from build123d import *

# Parameters (mm, degrees)
SKETCH1_W              = 44
SKETCH1_H              = 320
BASE_FLANGE1_DEPTH     = 1.2
SKETCHED_START         = -22
SKETCHED_BEND1_DEPTH   = 44
SKETCHED_BEND1_2_DEPTH = 44
SKETCH7_R              = 4.5
CUT_EXTRUDE1_DEPTH     = 10
SKETCH8_R              = 4
CUT_EXTRUDE2_DEPTH     = 10


# Read off the part's stored shape, not the designer's step: Sketched Bend1
# Sheet-metal steps are written as plain solids
with BuildPart() as part:
    # Sketch1 → Base-Flange1 (new body)
    with BuildSketch(Plane(origin=(0, 0, 0), x_dir=(1, 0, 0), z_dir=(0, 1, 0))):
        Rectangle(SKETCH1_W, SKETCH1_H)
    extrude(amount=-BASE_FLANGE1_DEPTH)

    # Sketched Bend1 outline → Sketched Bend1 (cut)
    with BuildSketch(Plane.YZ.offset(SKETCHED_START)):
        with BuildLine():
            Line((0, -160), (0, -65.054444388))
            ThreePointArc((0, -65.054444388), (-0.872269031, -64.341342484), (-1.2, -63.2634))
            Line((-1.2, -63.2634), (-1.2, -160))
            Line((-1.2, -160), (0, -160))
        make_face()
    extrude(amount=SKETCHED_BEND1_DEPTH, mode=Mode.SUBTRACT)

    # Sketched Bend1 2 outline → Sketched Bend1 2 (add)
    with BuildSketch(Plane.YZ.offset(SKETCHED_START)):
        with BuildLine():
            Line((93.6, -64), (0.7366, -64))
            ThreePointArc((0.7366, -64), (0.215745145, -63.784254855), (0, -63.2634))
            Line((0, -63.2634), (0, -65.054444388))
            ThreePointArc((0, -65.054444388), (0.361178238, -65.163262642), (0.7366, -65.2))
            Line((0.7366, -65.2), (93.6, -65.2))
            Line((93.6, -65.2), (93.6, -64))
        make_face()
    extrude(amount=SKETCHED_BEND1_2_DEPTH)

    # Sketch7 → Cut-Extrude1 (cut)
    with BuildSketch(Plane(origin=(0, 0, -65.2), x_dir=(-1, 0, 0), z_dir=(0, 0, -1))):
        with Locations(Location((0, 73.6, 0), (0, 0, 90))):
            Circle(SKETCH7_R)
    extrude(amount=-CUT_EXTRUDE1_DEPTH, mode=Mode.SUBTRACT)

    # Sketch8 → Cut-Extrude2 (cut)
    with BuildSketch(Plane.XZ.offset(1.2)):
        with Locations(Location((0, 8.8, 0), (0, 0, 270))):
            Circle(SKETCH8_R)
        with Locations(Location((0, 148.8, 0), (0, 0, 270))):
            Circle(SKETCH8_R)
    extrude(amount=-CUT_EXTRUDE2_DEPTH, mode=Mode.SUBTRACT)


solid = part.part
Verification items for the finished model (mm, model axes). A direction names the side the tool comes from. Coordinates: 2 decimals unless noted, no trailing zeros. Write each loop counter-clockwise with the first axis right and the second up, starting at its lowest first coordinate (ties: lowest second). Pieces come first, ordered by that corner, then holes. Notation, with made-up numbers: (-7, 73) - (50, 73) arc R16 cw to (50, 96) - close; hole circle Ø11 at (17.5, 44). An arc over 180 degrees is marked (long way). Answer as a JSON object with one key per item and string values.
(1) Cross-section at C-C on x = -8.5. Record the cut outline in (y, z), plus the area to 3 significant figures.
Report:
{"outline": "(-1.2, -63.26) arc R1.94 ccw to (0.74, -65.2) - (93.6, -65.2) - (93.6, -64) - (0.74, -64) arc R0.74 cw to (0, -63.26) - (0, 160) - (-1.2, 160) - close", "area": "382 mm^2"}
(2) Cross-section at A-A on z = 8.8. Record the cut outline in (x, y).
Report:
{"outline": "(-22, -1.2) - (-4, -1.2) - (-4, 0) - (-22, 0) - close; (4, -1.2) - (22, -1.2) - (22, 0) - (4, 0) - close"}
(3) Cross-section at B-B on y = 73.6. Record the cut outline in (x, z).
Report:
{"outline": "(-22, -65.2) - (-4.5, -65.2) - (-4.5, -64) - (-22, -64) - close; (4.5, -65.2) - (22, -65.2) - (22, -64) - (4.5, -64) - close"}
(4) Tool access check on faces 4 (the flat face through (0, 47, -65.2)), 5 (the flat face through (0, 0, 47)). Record the directions out of +Z, -Z, +X, -X, +Y, -Y that give a thin tool (end or side, any length) a straight path to the whole face; none if there is none.
Report:
{"face 4": "-Z, +X, -X, +Y, -Y", "face 5": "+Z, +X, -X, +Y"}
(5) Mould release check, pull along Y, two halves, no side actions. Record for faces 1 (the cylindrical face through (0.176, -0.608, 152.796)), 2 (the cylindrical face through (0.198, 69.104, -64.608)), 3 (the flat face through (0, -1.2, 47)): pulls with the +Y half, pulls with the -Y half, needs draft (parallel to the pull), parting line crosses it, or undercut.
Report:
{"face 1": "needs draft", "face 2": "undercut", "face 3": "pulls with the -Y half"}
(6) Gauge pin test, flat ends, axial feed: pin 1 Ø13 at (x, z) = (0, 148.8) entering from +Y; pin 2 Ø8 at (x, y) = (13, 45.5) entering from +Z; pin 3 Ø5 at (x, z) = (0, 8.8) entering from -Y. Record the tip position at first contact, or that the pin passes through.
Report:
{"pin 1": "y = 0", "pin 2": "z = -64", "pin 3": "through"}
(7) Cross-section at D-D on y = 31.5. Record the cut outline in (x, z).
Report:
{"outline": "(-22, -65.2) - (22, -65.2) - (22, -64) - (-22, -64) - close"}
(8) Thickness scan on line 1 along X through (y, z) = (-0.75, 8.8); line 2 along Z through (x, y) = (3, 86); line 3 along Y through (x, z) = (9, -55). Record the ranges inside material, lowest first.
Report:
{"line 1": "-22 to -4, 4 to 22", "line 2": "-65.2 to -64", "line 3": "-1.2 to 0"}
